The listing builds one solid part. Answer for the finished solid, in the listing's coordinates (mm). Round coordinates to 2 decimals unless told otherwise and drop trailing zeros. Order: outer loops, then holes, each group sorted by start corner. A loop starts at its lowest first (then second) coordinate and runs counter-clockwise, first axis right, second up. Notation, with made-up numbers: (45, 24.5) -> (70, 24.5) arc R26 ccw to (70, 50.5) -> close; hole circle Ø9 at (26, 34.5). An arc over 180 degrees is marked (long way). Answer in a Markdown table with one row per item. Add a question column.
```python
from build123d import *

# Parameters (mm, degrees)
BOSS_EXTRU_1_DEPTH      = 1.524
CONG_1_R                = 4.318
BOSS_EXTRU_3_START      = -1.524
BOSS_EXTRU_3_DEPTH      = 1.524
ESQUISSE3_R             = 2
ENL_V_MAT_EXTRU_1_DEPTH = 127.347243097


with BuildPart() as part:
    # Esquisse1 → Boss.-Extru.1 (new body)
    with BuildSketch(Plane(origin=(0, 0, 0), x_dir=(1, 0, 0), z_dir=(0, 1, 0))):
        with BuildLine():
            Line((-95.25, 0), (95.25, 0))
            ThreePointArc((95.25, 0), (0, 83.82), (-95.25, 0))
        make_face()
    extrude(amount=BOSS_EXTRU_1_DEPTH)

    # Congé1
    cong_1_edges = [part.edges().sort_by_distance(p)[0] for p in [
        (-95.25, 0.762, 0),
        (95.25, 0.762, 0),
    ]]
    fillet(cong_1_edges, radius=CONG_1_R)

    # Esquisse2 → Boss.-Extru.3 (add)
    with BuildSketch(Plane(origin=(0, 1.524, 0), x_dir=(1, 0, 0), z_dir=(0, 1, 0)).offset(BOSS_EXTRU_3_START)):
        with BuildLine():
            ThreePointArc((62.546228877, 60.657678488), (63.115798852, 69.065741324), (55.110603719, 66.431964286))
            ThreePointArc((55.110603719, 66.431964286), (58.899220354, 63.635996718), (62.546228877, 60.657678488))
        make_face()
        with BuildLine():
            ThreePointArc((-62.546228877, 60.657678488), (-58.899220354, 63.635996718), (-55.110603719, 66.431964286))
            ThreePointArc((-55.110603719, 66.431964286), (-63.115798852, 69.065741324), (-62.546228877, 60.657678488))
        make_face()
    extrude(amount=BOSS_EXTRU_3_DEPTH)

    # Esquisse3 → Enlèv. mat.-Extru.1 (cut, through all)
    with BuildSketch(Plane(origin=(0, 1.524, 0), x_dir=(1, 0, 0), z_dir=(0, 1, 0))):
        with Locations(Location((60, 4.445, 0), (0, 0, 270))):
            Circle(ESQUISSE3_R)
        with Locations(Location((-60, 4.445, 0), (0, 0, 270))):
            Circle(ESQUISSE3_R)
        with Locations(Location((-60, 65.445, 0), (0, 0, 270))):
            Circle(ESQUISSE3_R)
        with Locations(Location((60, 65.445, 0), (0, 0, 270))):
            Circle(ESQUISSE3_R)
    extrude(amount=-ENL_V_MAT_EXTRU_1_DEPTH, mode=Mode.SUBTRACT)


solid = part.part
```
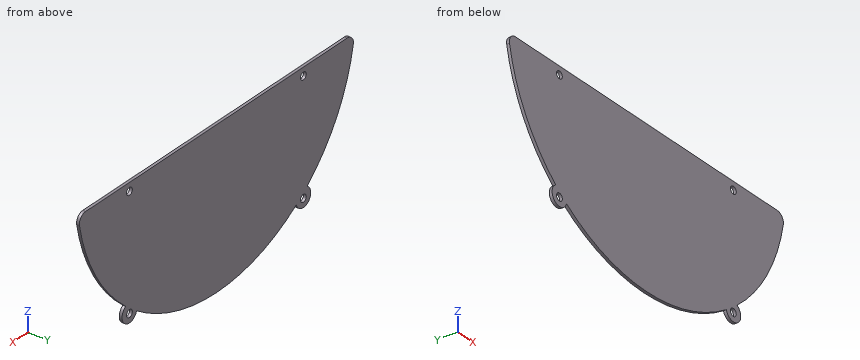
1. The part is cut by section B-B (x = -60). Give the vertices of the cut face in (y, z) (3 decimals).
2. The part is cut by section A-A (y = 0.4). Give the vertices of the cut face in (x, z) (3 decimals).
3. The part is cut by section D-D (z = -24.5). Give the vertices of the cut face in (x, y), then the cut area to 3 significant figures.
4. The part is cut by section C-C (x = -39.5). Give the vertices of the cut face in (y, z), then the cut area to 3 significant figures.
5. Straight lines are drawn through the part: line 1 along X through (y, z) = (0.4, -76.5); line 2 along X through (y, z) = (0.5, -36.5); line 3 along Z through (x, y) = (71.5, 0.15). For each, find the intervals that lie inside material, in ascending order.
Report:
| question | item | result |
|---|---|---|
| 1 | outline | (0, -70.133) -> (1.524, -70.133) -> (1.524, -67.445) -> (0, -67.445) -> close; (0, -63.445) -> (1.524, -63.445) -> (1.524, -6.445) -> (0, -6.445) -> close; (0, -2.445) -> (1.524, -2.445) -> (1.524, 0) -> (0, 0) -> close |
| 2 | outline | (-94.457, -5.096) arc R96.029 ccw to (-62.546, -60.658) arc R5.08 ccw (long way) to (-55.111, -66.432) arc R96.029 ccw to (55.111, -66.432) arc R5.08 ccw (long way) to (62.546, -60.658) arc R96.029 ccw to (94.457, -5.096) arc R4.318 ccw to (90.21, 0) -> (-90.21, 0) arc R4.318 ccw to start; hole circle Ø4 at (-60, -65.445); hole circle Ø4 at (-60, -4.445); hole circle Ø4 at (60, -65.445); hole circle Ø4 at (60, -4.445) |
| 3 | outline | (-88.74, 0) -> (88.74, 0) -> (88.74, 1.52) -> (-88.74, 1.52) -> close |
| 3 | area | 270 mm^2 |
| 4 | outline | (0, -75.32) -> (1.52, -75.32) -> (1.52, 0) -> (0, 0) -> close |
| 4 | area | 115 mm^2 |
| 5 | line 1 | x = -36.77 to 36.77 |
| 5 | line 2 | x = -82.76 to 82.76 |
| 5 | line 3 | z = -51.9 to 0 |
